```python
from build123d import *

# Parameters (mm, degrees)
F1_DEPTH = 63.5
F0_W     = 25.4
F0_H     = 19.05
F2_DEPTH = 25.4
F3_DEPTH = 7.9375
F5_R     = 6.35


with BuildPart() as f1:
    # F0 (on Front) → F1 (new body, symmetric)
    with BuildSketch(Plane.XZ):
        Polygon((-41.275, 9.525), (-41.275, -9.525), (41.275, -9.525), (41.275, 9.525), (22.225, 9.525), align=None)
    extrude(amount=F1_DEPTH, both=True)

    # F0 (on Front) → F2 (join, symmetric)
    with BuildSketch(Plane.XZ):
        with Locations((73.025, 52.4002)):
            Rectangle(F0_W, F0_H)
        with BuildLine():
            Line((22.225, 9.525), (41.275, 9.525))
            Line((41.275, 9.525), (41.275, 27.0002))
            ThreePointArc((41.275, 27.0002), (45.9246798487, 38.2255201513), (57.15, 42.8752))
            Line((57.15, 42.8752), (60.325, 42.8752))
            Line((60.325, 42.8752), (60.325, 61.9252))
            Line((60.325, 61.9252), (57.15, 61.9252))
            add(Edge.make_bspline(
                [(54.4617401278, 61.8215854385), (55.3652962771, 61.8675171828), (56.2616391895, 61.9021368307), (57.15, 61.9252)],
                knots=[109.0694907263, 109.0694907263, 109.0694907263, 109.0694907263, 111.5045361635, 111.5045361635, 111.5045361635, 111.5045361635], degree=3))
            ThreePointArc((54.4617401278, 61.8215854385), (31.5214699891, 50.7264317801), (22.225, 27.0002))
            Line((22.225, 27.0002), (22.225, 9.525))
        make_face()
    extrude(amount=F2_DEPTH, both=True)

    # F0 (on Front) → F3 (join, symmetric)
    with BuildSketch(Plane.XZ):
        with BuildLine():
            add(Edge.make_bspline(
                [(-41.275, 9.525), (-40.9534464322, 35.0115971257), (13.9900480858, 59.7642308284), (54.4617401278, 61.8215854385)],
                knots=[0, 0, 0, 0, 109.0694907263, 109.0694907263, 109.0694907263, 109.0694907263], degree=3))
            Line((-41.275, 9.525), (22.225, 9.525))
            Line((22.225, 9.525), (22.225, 27.0002))
            ThreePointArc((22.225, 27.0002), (31.5214699891, 50.7264317801), (54.4617401278, 61.8215854385))
        make_face()
    extrude(amount=F3_DEPTH, both=True)

    # F0 (on Front) → F4 (revolve)
    with BuildSketch(Plane.XZ):
        Polygon((85.725, 66.675), (85.725, 61.9252), (85.725, 42.8752), (85.725, 38.1), (111.125, 38.1), (111.125, 66.675), align=None)
    revolve(axis=Axis((85.725, 0, 52.3875), (0, 0, 1)))

    # F5
    f5_edges = [f1.edges().sort_by_distance(p)[0] for p in [
        (41.275, -63.5, 0),
        (-41.275, -63.5, 0),
        (-41.275, 63.5, 0),
        (41.275, 63.5, 0),
    ]]
    fillet(f5_edges, radius=F5_R)


solid = f1.part
```
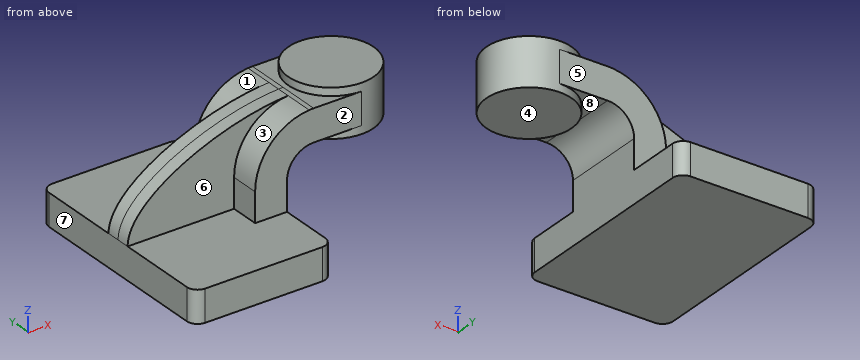
Geometry: final body of the model. Coordinates: model frame, mm. Face numbers are marked on the shaded views. A direction names the side the tool comes from. Round coordinates to 2 decimals unless told otherwise and drop trailing zeros. Write each loop counter-clockwise with the first axis right and the second up, starting at its lowest first coordinate (ties: lowest second). Pieces come first, ordered by that corner, then holes. Notation, with made-up numbers: M 89,76.5 L 142,76.5 A25 cw 142,97.5 Z; hole C -19.75,3 d8. An arc over 180 degrees is marked long. Answer in a Markdown table with one row per item. Add a question column.
(1) Contact query for flat-ended pins moving along their axis: pin 1 (10 mm diameter, centred on y = 9.5, z = 30, fed in from +X); pin 2 (6 mm diameter, centred on x = 63, y = -19, fed in from +Z); pin 3 (8 mm diameter, centred on y = -4, z = 28.5, fed in from -X); pin 4 (10 mm diameter, centred on y = -33, z = 44.5, fed in from +X). Output: stop coordinate, or through.
(2) Ray query, L1, parallel to X at y = -16.5, z = -1.5 (3 decimals); L2, parallel to Z at x = -14.5, y = -57 (3 decimals); L3, parallel to X at y = 19, z = 27.5. Return the intervals inside material, ascending.
(3) Draft query along X for the marked faces 6, 7 and 8. Return one class per face: pulls with the +X half, pulls with the -X half, needs draft (parallel to the pull), parting line crosses it, or undercut.
(4) Cut plane B-B, the plane y = 29. Return the cut outline in (x, z) (3 decimals), then the cut area to 3 significant figures.
(5) Cut plane A-A, the plane z = -2. Return the cut outline in (x, y) (3 decimals), then the cut area to 3 significant figures.
(6) Reachability of the marked faces 1, 2, 3, 4 and 5 from +Z, -Z, +X, -X, +Y, -Y: full face, straight path, thin tool, end or side. Return the list, or none.
Established:
| question | item | result |
|---|---|---|
| 1 | pin 1 | x = 43.44 |
| 1 | pin 2 | z = 61.93 |
| 1 | pin 3 | x = -35.12 |
| 1 | pin 4 | through |
| 2 | L1 | -41.275 to 41.275 |
| 2 | L2 | -9.525 to 9.525 |
| 2 | L3 | 22.23 to 41.28 |
| 3 | face 6 | needs draft |
| 3 | face 7 | pulls with the -X half |
| 3 | face 8 | undercut |
| 4 | outline | M -41.275,-9.525 L 41.275,-9.525 L 41.275,9.525 L -41.275,9.525 Z |
| 4 | area | 1,570 mm² |
| 5 | outline | M -41.275,-57.15 A6.35 ccw -34.925,-63.5 L 34.925,-63.5 A6.35 ccw 41.275,-57.15 L 41.275,57.15 A6.35 ccw 34.925,63.5 L -34.925,63.5 A6.35 ccw -41.275,57.15 Z |
| 5 | area | 10,400 mm² |
| 6 | face 1 | +Z, -X, +Y |
| 6 | face 2 | +Z, +X, -X, -Y |
| 6 | face 3 | +Z, -X, -Y |
| 6 | face 4 | -Z, +X, +Y, -Y |
| 6 | face 5 | +Z, +X, -X, +Y |
